from build123d import *

# Parameters (mm, degrees)
PAD_DEPTH    = 2.5
SKETCH001_R  = 1.6
SKETCH001_W  = 30.35
SKETCH001_H  = 12.35
POCKET_DEPTH = 5
SKETCH002_W  = 1
SKETCH002_H  = 18
PAD001_DEPTH = 4
FILLET_R     = 5


with BuildPart() as part:
    # Sketch → Pad (new body)
    with BuildSketch(Plane.XY):
        Polygon((-69, 9), (21, 9), (21, 22), (69, 22), (69, 10.0438), (69, -9), (-69, -9), align=None)
    extrude(amount=PAD_DEPTH)

    # Sketch001 → Pocket (cut)
    with BuildSketch(Plane.XY.offset(2.5)):
        with Locations((-64.5, 0)):
            Circle(SKETCH001_R)
        with Locations((27, 13)):
            Circle(SKETCH001_R)
        with Locations((63, 13)):
            Circle(SKETCH001_R)
        with Locations((45, 13)):
            Rectangle(SKETCH001_W, SKETCH001_H)
    extrude(amount=-POCKET_DEPTH, mode=Mode.SUBTRACT)

    # Sketch002 → Pad001 (new body)
    with BuildSketch(Plane(origin=(0, 0, 0), x_dir=(1, 0, 0), z_dir=(0, 0, -1))):
        with Locations((-59.5, 0)):
            Rectangle(SKETCH002_W, SKETCH002_H)
    extrude(amount=PAD001_DEPTH)

    # Fillet
    fillet_edges = [part.edges().sort_by_distance(p)[0] for p in [
        (69, 22, 1.25),
        (21, 22, 1.25),
        (69, -9, 1.25),
    ]]
    fillet(fillet_edges, radius=FILLET_R)


solid = part.part
The listing builds one solid part. Answer for the finished solid, in the listing's coordinates (mm). A direction names the side the tool comes from. Give positions to 0.01 mm unless a question says otherwise; leave off trailing zeros. Loops run counter-clockwise (first coordinate to the right, second up) from the corner with the lowest first, then second, coordinate; pieces in that order, holes last. Notation, with made-up numbers: (28.5, 86) - (81.5, 86) arc R29 ccw to (81.5, 122) - close; hole circle Ø11 at (73, 15.5). An arc over 180 degrees is marked (long way). Write each question's results on one line, items separated by ' | '.
1. Find section B-B, the plane y = 0. Write down the section's boundary in (x, z), then the cut area to 3 significant figures.
Resolved:
outline: (-69, 0) - (-66.1, 0) - (-66.1, 2.5) - (-69, 2.5) - close; (-62.9, 0) - (-60, 0) - (-60, -4) - (-59, -4) - (-59, 0) - (69, 0) - (69, 2.5) - (-62.9, 2.5) - close | area: 341 mm^2
2. Which of the six approach directions +Z, -Z, +X, -X, +Y, -Y give full straight-line access (tool end or side, diameter ignored) to faces 1 (the face through (21, 13, 1)), 2 (the face through (-59, 0, -2)), 3 (the face through (45, 19.175, 1))?
Resolved:
face 1: +Z, -Z, -X, +Y | face 2: -Z, +X, +Y, -Y | face 3: +Z, -Z
3. Find section A-A, the plane x = 47. Write down the section's boundary in (y, z) (3 decimals), then the cut area to 3 significant figures.
Resolved:
outline: (-9, 0) - (6.825, 0) - (6.825, 2.5) - (-9, 2.5) - close; (19.175, 0) - (22, 0) - (22, 2.5) - (19.175, 2.5) - close | area: 46.6 mm^2
4. Flat-ended cylindrical pins translate along their axes: P1, Ø1.2, axis at y = 15.5, z = 2, coming from the -X side; P2, Ø2, axis at y = -2, z = -2.5, coming from the -X side; P3, Ø5, axis at x = 27, y = 13, coming from the -Z side. Find the tip coordinate at first contact, or state that the pin passes through.
Resolved:
P1: stops at x = 21 | P2: stops at x = -60 | P3: stops at z = 0
5. For a pull along Y with two mould halves and no side action, classify faces 4 (the face through (45, 6.825, 1)), 5 (the face through (-2, -9, 1)), 6 (the face through (60.175, 13, 1)), 7 (the face through (22, 20, 1)) as +Y half, -Y half, draft (parallel to the pull), parting line (faces both ways), or undercut.
Resolved:
face 4: undercut | face 5: -Y half | face 6: undercut | face 7: +Y half
6. Find section D-D, the plane x = -64.5. Write down the section's boundary in (y, z).
Resolved:
outline: (-9, 0) - (-1.6, 0) - (-1.6, 2.5) - (-9, 2.5) - close; (1.6, 0) - (9, 0) - (9, 2.5) - (1.6, 2.5) - close
7. Find section C-C, the plane z = 1.25. Write down the section's boundary in (x, y) (3 decimals), then the cut area to 3 significant figures.
Resolved:
outline: (-69, -9) - (64, -9) arc R5 ccw to (69, -4) - (69, 17) arc R5 ccw to (64, 22) - (26, 22) arc R5 ccw to (21, 17) - (21, 9) - (-69, 9) - close; hole circle Ø3.2 at (-64.5, 0); hole circle Ø3.2 at (27, 13); hole (29.825, 6.825) - (60.175, 6.825) - (60.175, 19.175) - (29.825, 19.175) - close; hole circle Ø3.2 at (63, 13) | area: 2,690 mm^2
8. Consider probe 1 along Y at (x, z) = (-64.5, 1.55); probe 2 along Y at (x, z) = (27, 1.7); probe 3 along X at (y, z) = (12, 1.5) (3 decimals). Determine where each line is inside the solid, lowest interval first. Write a range as from..to.
Resolved:
probe 1: y = -9..-1.6, 1.6..9 | probe 2: y = -9..11.4, 14.6..22 | probe 3: x = 21..25.751, 28.249..29.825, 60.175..61.751, 64.249..69
